from build123d import *

# Parameters (mm, degrees)
SKETCH1_W                                       = 400
SKETCH1_H                                       = 305
BOSS_EXTRUDE1_DEPTH                             = 12
CBORE_FOR_M5_SOCKET_HEAD_CAP_SCREW1_D           = 5.5
CBORE_FOR_M5_SOCKET_HEAD_CAP_SCREW1_CBORE_D     = 10
CBORE_FOR_M5_SOCKET_HEAD_CAP_SCREW1_CBORE_DEPTH = 5
M5X0_8_TAPPED_HOLE1_D                           = 4.2
M5X0_8_TAPPED_HOLE1_DEPTH                       = 14
M5X0_8_TAPPED_HOLE1_TIP                         = 1.2618073
CHAMFER1_SIZE                                   = 10
M8_CLEARANCE_HOLE1_D                            = 9
M5X0_8_TAPPED_HOLE2_D                           = 4.2


with BuildPart() as part:
    # Sketch1 → Boss-Extrude1 (new body)
    with BuildSketch(Plane(origin=(0, 0, 0), x_dir=(1, 0, 0), z_dir=(0, 1, 0))):
        with Locations((0, -152.5)):
            Rectangle(SKETCH1_W, SKETCH1_H)
    extrude(amount=BOSS_EXTRUDE1_DEPTH)

    # CBORE for M5 Socket Head Cap Screw1 (through all)
    with Locations(Plane.XZ):
        with Locations((-9, 230), (-9, 70), (9, 70), (9, 230)):
            CounterBoreHole(CBORE_FOR_M5_SOCKET_HEAD_CAP_SCREW1_D / 2, CBORE_FOR_M5_SOCKET_HEAD_CAP_SCREW1_CBORE_D / 2, CBORE_FOR_M5_SOCKET_HEAD_CAP_SCREW1_CBORE_DEPTH)

    # M5x0.8 Tapped Hole1
    with Locations(Plane.XY.offset(305)):
        with Locations((-38, 6), (12, 6)):
            Hole(M5X0_8_TAPPED_HOLE1_D / 2, depth=M5X0_8_TAPPED_HOLE1_DEPTH)
            with Locations((0, 0, -(M5X0_8_TAPPED_HOLE1_DEPTH + M5X0_8_TAPPED_HOLE1_TIP / 2))):  # 118° drill point
                Cone(0, M5X0_8_TAPPED_HOLE1_D / 2, M5X0_8_TAPPED_HOLE1_TIP, mode=Mode.SUBTRACT)

    # Chamfer1
    chamfer1_edges = [part.edges().sort_by_distance(p)[0] for p in [
        (-200, 6, 0),
        (200, 6, 0),
        (200, 6, 305),
        (-200, 6, 305),
    ]]
    chamfer(chamfer1_edges, length=CHAMFER1_SIZE)

    # M8 Clearance Hole1 (through all)
    with Locations(Plane(origin=(0, 12, 0), x_dir=(-1, 0, 0), z_dir=(0, 1, 0))):
        with Locations((185, 290), (185, 15), (-185, 15), (-185, 290)):
            Hole(M8_CLEARANCE_HOLE1_D / 2)

    # M5x0.8 Tapped Hole2 (through all)
    with Locations(Plane(origin=(0, 12, 0), x_dir=(-1, 0, 0), z_dir=(0, 1, 0))):
        with Locations((51, 265), (51, 35), (-110, 265), (-110, 35)):
            Hole(M5X0_8_TAPPED_HOLE2_D / 2)


solid = part.part
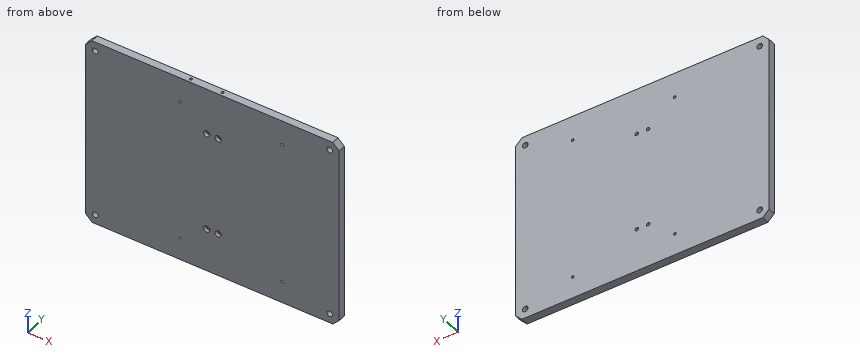
The listing builds one solid part. Answer for the finished solid, in the listing's coordinates (mm). Round coordinates to 2 decimals unless told otherwise and drop trailing zeros. Loops run counter-clockwise (first coordinate to the right, second up) from the corner with the lowest first, then second, coordinate; pieces in that order, holes last. Notation, with made-up numbers: M 12.25,53 L 25.25,53 A35 cw 25.25,91 Z; hole C -12,21.5 d8. An arc over 180 degrees is marked long. Return JSON: item names as keys, results as strings.
Q1. Find the intervals of material crossed by line 1 along Z through (x, y) = (185, 8.25); line 2 along Z through (x, y) = (9, 1.7); line 3 along X through (y, z) = (7, 230), in increasing order. Write a range as from..to.
Results list:
{"line 1": "z = 0..10.5, 19.5..285.5, 294.5..305", "line 2": "z = 0..65, 75..225, 235..305", "line 3": "x = -200..-11.75, -6.25..6.25, 11.75..200"}
Q2. Find section A-A, the plane x = -185. Determine the outline of the cut face in (y, z).
Results list:
{"outline": "M 0,0 L 12,0 L 12,10.5 L 0,10.5 Z; M 0,19.5 L 12,19.5 L 12,285.5 L 0,285.5 Z; M 0,294.5 L 12,294.5 L 12,305 L 0,305 Z"}
Q3. This flat-tipped pin is pushed along its axis until it touches: pin 1 Ø8 at (x, z) = (9, 70) entering from -Y. Where does it stop, or does it pass through?
Results list:
{"pin 1": "stops at y = 5"}
